Geometry check sheet. Reference: drawing and pictorial views, mm from the part's lowest x, y, z. Give positions to 0.01 mm unless a question says otherwise; leave off trailing zeros. Loops run counter-clockwise (first coordinate to the right, second up) from the corner with the lowest first, then second, coordinate; pieces in that order, holes last. Notation, with made-up numbers: (57.25, -25.75) - (89.25, -25.75) arc R15 ccw to (89.25, -21.75) - close; hole circle Ø3 at (10.5, 89.25). An arc over 180 degrees is marked (long way). Put each result on its own line as item: value. Start each with the question number.
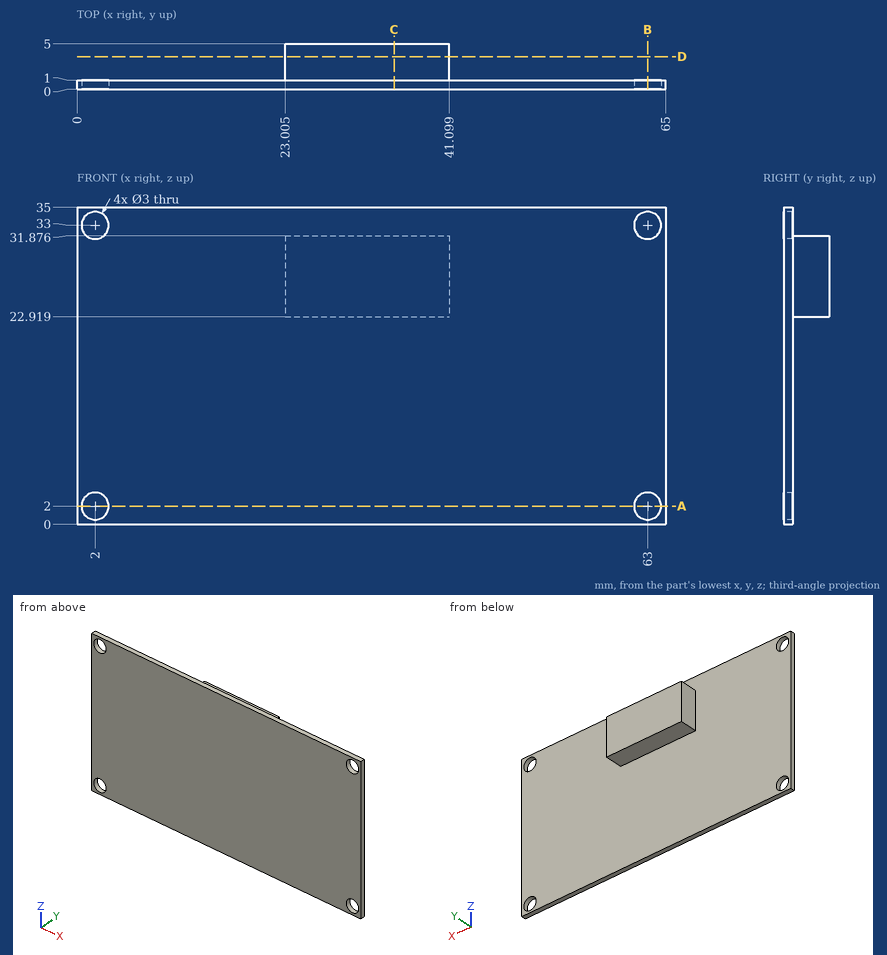
1) Section check D-D, the plane y = 3.6. Enter the section's corners in (x, z) (1 decimal).
2) Section check B-B, the plane x = 63. Enter the section's corners in (y, z).
3) Section check C-C, the plane x = 35. Enter the section's corners in (y, z).
4) Section check A-A, the plane z = 2. Enter the section's corners in (x, y).
5) Scan lines: line 1 along Z through (x, y) = (63, 0.5); line 2 along X through (y, z) = (0.6, 33); line 3 along Z through (x, y) = (38, 4.2). Record each from-to range of solid material in increasing order. Write a range as from..to.
6) Depth check by flat-ended pin: P1, Ø1, axis at x = 58, z = 11.5, coming from the +Y side; P2, Ø3.5, axis at x = 2, z = 2, coming from the -Y side; P3, Ø1.2, axis at y = 2.5, z = 26.5, coming from the +X side; P4, Ø3, axis at x = 28.5, y = 3, coming from the +Z side. Enter the tip coordinate at first touch or a pass-through.
Results are:
1. outline: (23, 22.9) - (41.1, 22.9) - (41.1, 31.9) - (23, 31.9) - close
2. outline: (0, 0) - (1, 0) - (1, 0.5) - (0, 0.5) - close; (0, 3.5) - (1, 3.5) - (1, 31.5) - (0, 31.5) - close; (0, 34.5) - (1, 34.5) - (1, 35) - (0, 35) - close
3. outline: (0, 0) - (1, 0) - (1, 22.92) - (5, 22.92) - (5, 31.88) - (1, 31.88) - (1, 35) - (0, 35) - close
4. outline: (0, 0) - (0.5, 0) - (0.5, 1) - (0, 1) - close; (3.5, 0) - (61.5, 0) - (61.5, 1) - (3.5, 1) - close; (64.5, 0) - (65, 0) - (65, 1) - (64.5, 1) - close
5. line 1: z = 0..0.5, 3.5..31.5, 34.5..35
5. line 2: x = 0..0.5, 3.5..61.5, 64.5..65
5. line 3: z = 22.92..31.88
6. P1: stops at y = 1
6. P2: stops at y = 0
6. P3: stops at x = 41.1
6. P4: stops at z = 31.88
